Autodesk Fusion 360 part; units mm, degrees
sketch "Sketch1" plane through (0, 0, 0) normal (0, 0, 1) x (1, 0, 0)
  circle A0 centre (0, 0) radius 2.85
  dimension "d1" = 5.7
extrude "Extrude1" add sketch "Sketch1" along normal blind 1.65
fillet "Fillet1" radius 1 1 edges at (-2.6571, -1.0306, 1.65)
sketch "Sketch2" plane through (0, 0, 1.65) normal (0, 0, 1) x (1, 0, 0)
  circle A0 centre (0, 0) radius 1.85
  line L0 (-0.641, 1.131) -> (-1.3, 0.0104)
  line L1 (-1.3, 0.0104) -> (-0.659, -1.1206)
  line L2 (-0.659, -1.1206) -> (0.641, -1.131)
  line L3 (0.641, -1.131) -> (1.3, -0.0104)
  line L4 (1.3, -0.0104) -> (0.659, 1.1206)
  line L5 (0.659, 1.1206) -> (-0.641, 1.131)
  dimension "d6" = 1.3
extrude "Extrude2" cut sketch "Sketch2" against normal blind 1 contours L0 L1 L2 L3 L4 L5
sketch "Sketch3" plane through (0, 0, 0) normal (0, 0, -1) x (-1, 0, 0)
  circle A0 centre (0, 0) radius 2.85
  circle A1 centre (0, 0) radius 1.5
  dimension "d9" = 3
extrude "Extrude3" add sketch "Sketch3" along normal blind 12 contours A1
Input: part model. Units: mm. Frame: model coordinates. A direction names the side the tool comes from. Give positions to 0.01 mm unless a question says otherwise; leave off trailing zeros. Order: outer loops, then holes, each group sorted by start corner. A loop starts at its lowest first (then second) coordinate and runs counter-clockwise, first axis right, second up.
1. Reachability of faces 5 (the flat face through (-1, -1, 1.65)), 6 (the flat face through (0, 0, 0.65)), 7 (the flat face through (1.2, -1.2, 0)) from +Z, -Z, +X, -X, +Y, -Y: full face, straight path, thin tool, end or side. Return the list, or none.
Derived:
face 5: +Z, +X, -X, +Y, -Y
face 6: +Z
face 7: -Z
2. Mould query, pull axis Y, two halves, no side actions, for faces 1 (the flat face through (-0.984, -0.547, 1.157)), 2 (the flat face through (0, 0, -12)), 3 (the flat face through (0.966, -0.579, 1.157)), 4 (the cylindrical face through (-2.262, 1.734, 0.32)). Classes: released by +Y, released by -Y, zero draft, split by the parting line, or undercut.
Derived:
face 1: undercut
face 2: zero draft
face 3: undercut
face 4: split by the parting line
3. Pin query (flat end, axial travel): pin 1 (3 mm diameter, centred on x = -1.5, y = 1, fed in from -Z); pin 2 (1.5 mm diameter, centred on x = 1, z = -3.5, fed in from +Y); pin 3 (0.7 mm diameter, centred on x = -0.5, y = 0, fed in from +Z); pin 4 (1 mm diameter, centred on y = -1, z = -2, fed in from -X). Return the tip coordinate at first contact, or that it passes through.
Derived:
pin 1: stops at z = -12
pin 2: stops at y = 1.48
pin 3: stops at z = 0.65
pin 4: stops at x = -1.41
4. Section A-A on x = 0. Return the cut outline in (y, z), and give its area (3 significant figures).
Derived:
outline: (-2.85, 0) - (-1.5, 0) - (-1.5, -12) - (1.5, -12) - (1.5, 0) - (2.85, 0) - (2.85, 0.65) arc R1 ccw to (1.85, 1.65) - (1.13, 1.65) - (1.13, 0.65) - (-1.13, 0.65) - (-1.13, 1.65) - (-1.85, 1.65) arc R1 ccw to (-2.85, 0.65) - close
area: 42.7 mm2
5. Material intervals for L1, parallel to X at y = -0.75, z = -0.25; L2, parallel to Z at x = -1.45, y = 0.5; L3, parallel to Y at x = 1, z = -6, sorted ascending.
Derived:
L1: x = -1.3 to 1.3
L2: z = 0 to 1.65
L3: y = -1.12 to 1.12
6. Section B-B on z = -7. Return the cut outline in (x, y), and give its area (3 significant figures).
Derived:
outline: circle Ø3 at (0, 0)
area: 7.07 mm2
